```python
from build123d import *

# Parameters (mm, degrees)
SKETCH1_W           = 2.2
SKETCH1_H           = 4.7
BOSS_EXTRUDE1_DEPTH = 2
SKETCH2_W           = 4.6
SKETCH2_H           = 7.1
SKETCH2_W_2         = 2.2
SKETCH2_H_2         = 4.7
BOSS_EXTRUDE2_DEPTH = 20
SKETCH3_W           = 2.2
SKETCH3_H           = 4.7
BOSS_EXTRUDE3_DEPTH = 1
SKETCH5_R           = 1.35
BOSS_EXTRUDE4_DEPTH = 8
FILLET1_R           = 2
SKETCH6_W           = 1.9
SKETCH6_H           = 7.433939444
BOSS_EXTRUDE5_DEPTH = 8


with BuildPart() as part:
    # Sketch1 → Boss-Extrude1 (new body)
    with BuildSketch(Plane.XY):
        Polygon((49, 70), (39, 70), (39, 58.55), (33.2, 58.55), (33.2, 51.45), (39, 51.45), (39, 40), (49, 40), align=None)
        with Locations((35.5, 55)):
            Rectangle(SKETCH1_W, SKETCH1_H, mode=Mode.SUBTRACT)
    extrude(amount=BOSS_EXTRUDE1_DEPTH)

    # Sketch2 → Boss-Extrude2 (add)
    with BuildSketch(Plane(origin=(0, 0, 0), x_dir=(-1, 0, 0), z_dir=(0, 0, -1))):
        with Locations((-35.5, 55)):
            Rectangle(SKETCH2_W, SKETCH2_H)
        with Locations((-35.5, 55)):
            Rectangle(SKETCH2_W_2, SKETCH2_H_2, mode=Mode.SUBTRACT)
    extrude(amount=BOSS_EXTRUDE2_DEPTH)

    # Sketch3 → Boss-Extrude3 (add)
    with BuildSketch(Plane(origin=(0, 0, -20), x_dir=(-1, 0, 0), z_dir=(0, 0, -1))):
        with Locations((-35.5, 55)):
            Rectangle(SKETCH3_W, SKETCH3_H)
    extrude(amount=-BOSS_EXTRUDE3_DEPTH)

    # Sketch5 → Boss-Extrude4 (add)
    with BuildSketch(Plane(origin=(0, 0, 0), x_dir=(-1, 0, 0), z_dir=(0, 0, -1))):
        with Locations((-44, 45)):
            Circle(SKETCH5_R)
        with Locations((-44, 65)):
            Circle(SKETCH5_R)
    extrude(amount=BOSS_EXTRUDE4_DEPTH)

    # Fillet1
    fillet1_edges = [part.edges().sort_by_distance(p)[0] for p in [
        (49, 70, 1),
    ]]
    fillet(fillet1_edges, radius=FILLET1_R)
    fillet1_2_edges = [part.edges().sort_by_distance(p)[0] for p in [
        (39, 70, 1),
    ]]
    fillet(fillet1_2_edges, radius=FILLET1_R)
    fillet1_3_edges = [part.edges().sort_by_distance(p)[0] for p in [
        (49, 40, 1),
    ]]
    fillet(fillet1_3_edges, radius=FILLET1_R)
    fillet1_4_edges = [part.edges().sort_by_distance(p)[0] for p in [
        (39, 58.55, 1),
    ]]
    fillet(fillet1_4_edges, radius=FILLET1_R)
    fillet1_5_edges = [part.edges().sort_by_distance(p)[0] for p in [
        (39, 40, 1),
    ]]
    fillet(fillet1_5_edges, radius=FILLET1_R)
    fillet1_6_edges = [part.edges().sort_by_distance(p)[0] for p in [
        (39, 51.45, 1),
    ]]
    fillet(fillet1_6_edges, radius=FILLET1_R)

    # Sketch6 → Boss-Extrude5 (add)
    with BuildSketch(Plane(origin=(0, 0, 0), x_dir=(-1, 0, 0), z_dir=(0, 0, -1))):
        with Locations((-38.75, 55)):
            Rectangle(SKETCH6_W, SKETCH6_H)
    extrude(amount=BOSS_EXTRUDE5_DEPTH)


solid = part.part
```
Can you work these out from the model? Positions are in its coordinate system, mm. A direction names the side the tool comes from. Round coordinates to 2 decimals unless told otherwise and drop trailing zeros. Loops run counter-clockwise (first coordinate to the right, second up) from the corner with the lowest first, then second, coordinate; pieces in that order, holes last. Notation, with made-up numbers: (14, 75.25) -> (51, 75.25) arc R19 ccw to (51, 86.25) -> close; hole circle Ø4 at (78, 59). An arc over 180 degrees is marked (long way). One line per item, written item: value. Start each with the question number.
1. If I drill on probe 1 along Y at (x, z) = (35, -5); probe 2 along X at (y, z) = (53, -8.75); probe 3 along Z at (x, y) = (47.75, 67.5), over which ranges is the centre line in solid material (lowest first)?
2. If we section it at C-C, the plane x = 44: Write out the boundary of the cut face in (y, z).
3. For pin 1 (1 mm diameter, centred on y = 44.5, z = 1, fed in from -X); pin 2 (1.4 mm diameter, centred on y = 56, z = -13, fed in from +X); pin 3 (2 mm diameter, centred on x = 46, y = 59.5, fed in from -Z); pin 4 (2 mm diameter, centred on x = 38.5, y = 53.5, fed in from -Z), each with a flat end and sliding along its axis, tell me the tip position at first contact or that it passes through.
4. For faces 5 (the flat face through (35, 51.45, -9)), 6 (the flat face through (39, 58.717, -4)), 7 (the flat face through (36.6, 55, -8)), 8 (the cylindrical face through (44.29, 43.68, -3.94)), 9 (the flat face through (37.8, 55, -14)), which set-ups out of +Z, -Z, +X, -X, +Y, -Y let a thin tool reach every point of the face, with its end or its side?
5. If we mould it in two halves opening along X, with no side actions, what happens to faces 1 (the cylindrical face through (39.57, 40.6, 1.01)), 2 (the cylindrical face through (48.43, 69.4, 1.01)), 3 (the flat face through (34.4, 55, -8)), 4 (the flat face through (39, 51.283, -4))? For each: pulls with the +X half, pulls with the -X half, needs draft (parallel to the pull), parting line crosses it, or undercut.
6. If we section it at B-B, the plane z = -12: Write out the boundary of the cut face in (x, y), then the cut area to 3 significant figures.
7. If we section it at D-D, the plane y = 65: Write out the boundary of the cut face in (x, z).
8. If we section it at A-A, the plane z = -0.75: Write out the boundary of the cut face in (x, y).
Calculated:
1. probe 1: y = 51.45 to 52.65, 57.35 to 58.55
1. probe 2: x = 33.2 to 34.4, 36.6 to 37.8
1. probe 3: z = 0 to 2
2. outline: (40, 0) -> (43.65, 0) -> (43.65, -8) -> (46.35, -8) -> (46.35, 0) -> (63.65, 0) -> (63.65, -8) -> (66.35, -8) -> (66.35, 0) -> (70, 0) -> (70, 2) -> (40, 2) -> close
3. pin 1: stops at x = 39
3. pin 2: stops at x = 37.8
3. pin 3: stops at z = 0
3. pin 4: stops at z = -20
4. face 5: +Z, -Z, -X, -Y
4. face 6: -Z, +X, -X, +Y
4. face 7: +Z
4. face 8: -Z
4. face 9: -Z, +X, +Y, -Y
5. face 1: pulls with the -X half
5. face 2: pulls with the +X half
5. face 3: undercut
5. face 4: needs draft
6. outline: (33.2, 51.45) -> (37, 51.45) arc R2 cw to (37.8, 51.28) -> (37.8, 58.72) arc R2 cw to (37, 58.55) -> (33.2, 58.55) -> close; hole (34.4, 52.65) -> (36.6, 52.65) -> (36.6, 57.35) -> (34.4, 57.35) -> close
6. area: 22.4 mm²
7. outline: (39, 0) -> (42.65, 0) -> (42.65, -8) -> (45.35, -8) -> (45.35, 0) -> (49, 0) -> (49, 2) -> (39, 2) -> close
8. outline: (33.2, 51.45) -> (37, 51.45) arc R2 cw to (37.8, 51.28) -> (39.7, 51.28) -> (39.7, 58.72) -> (37.8, 58.72) arc R2 cw to (37, 58.55) -> (33.2, 58.55) -> close; circle Ø2.7 at (44, 45); circle Ø2.7 at (44, 65); hole (34.4, 52.65) -> (36.6, 52.65) -> (36.6, 57.35) -> (34.4, 57.35) -> close
